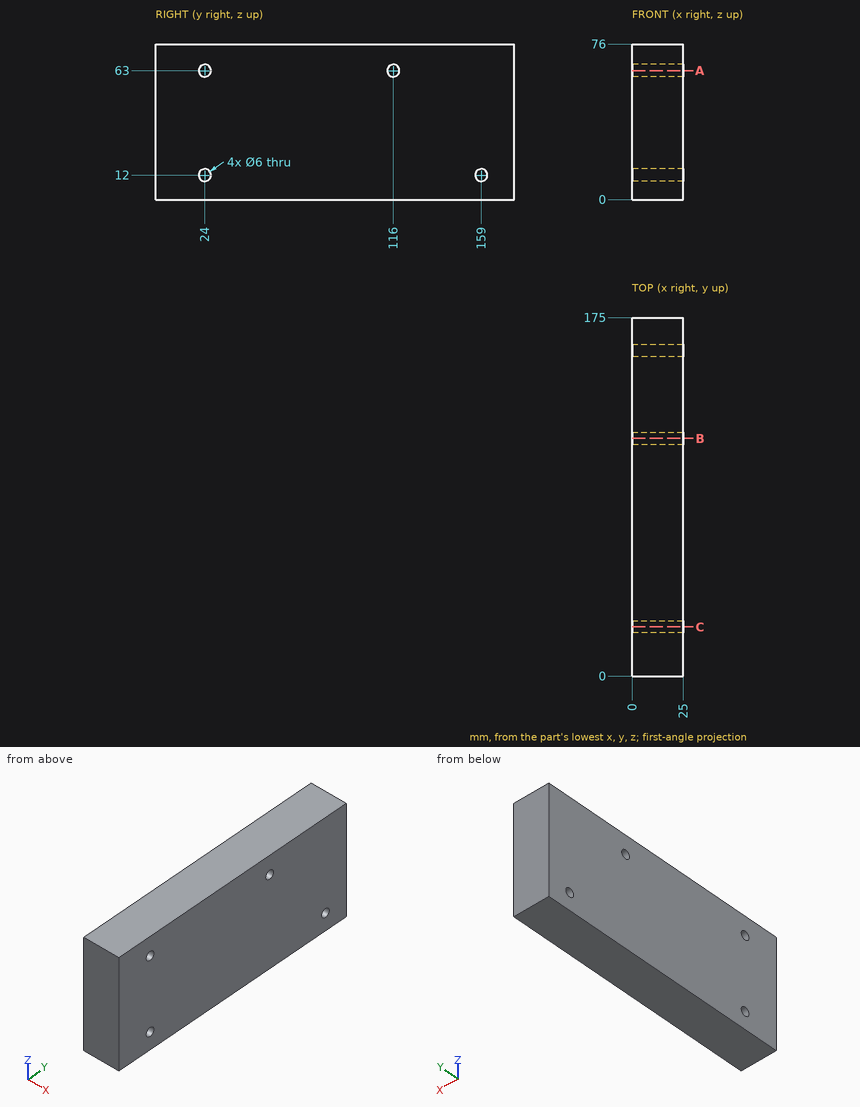
Geometry: see drawing. Coordinates: mm, zero at the bounding-box minimum. Give positions to 0.01 mm unless a question says otherwise; leave off trailing zeros. Order: outer loops, then holes, each group sorted by start corner. A loop starts at its lowest first (then second) coordinate and runs counter-clockwise, first axis right, second up. Notation, with made-up numbers: M 85,-28 L 123,-28 A30 ccw 123,5 Z; hole C -10.75,73.25 d3. An arc over 180 degrees is marked long. Answer as a JSON object with one key per item and string values.
1. Ray query, line 1 (Z direction, x = 7.75, y = 24); line 2 (Z direction, x = 6.5, y = 159); line 3 (Z direction, x = 11.75, y = 116). Return the intervals inside material, ascending. Write a range as [from, to].
Result sheet:
{"line 1": "[0, 9], [15, 60], [66, 76]", "line 2": "[0, 9], [15, 76]", "line 3": "[0, 60], [66, 76]"}
2. Cut plane C-C, the plane y = 24. Output: boundary loops of the cut face in (x, z).
Result sheet:
{"outline": "M 0,0 L 25,0 L 25,9 L 0,9 Z; M 0,15 L 25,15 L 25,60 L 0,60 Z; M 0,66 L 25,66 L 25,76 L 0,76 Z"}
3. Cut plane B-B, the plane y = 116. Output: boundary loops of the cut face in (x, z).
Result sheet:
{"outline": "M 0,0 L 25,0 L 25,60 L 0,60 Z; M 0,66 L 25,66 L 25,76 L 0,76 Z"}
4. Cut plane A-A, the plane z = 63. Output: boundary loops of the cut face in (x, y), and give its area (4 significant figures).
Result sheet:
{"outline": "M 0,0 L 25,0 L 25,21 L 0,21 Z; M 0,27 L 25,27 L 25,113 L 0,113 Z; M 0,119 L 25,119 L 25,175 L 0,175 Z", "area": "4,075 mm²"}
